The model under review builds one solid part; all positions refer to its coordinate system, in mm. A direction names the side the tool comes from. Give positions to 0.01 mm unless a question says otherwise; leave off trailing zeros. Order: outer loops, then holes, each group sorted by start corner. A loop starts at its lowest first (then second) coordinate and runs counter-clockwise, first axis right, second up. Notation, with made-up numbers: (-9.75, -30.5) - (6.25, -30.5) arc R18 cw to (6.25, -9.5) - close; hole circle Ø1 at (-7.5, 46). An arc over 180 degrees is marked (long way). Write item = value, one per line. Start each with the question number.
1. We need section A-A, the plane z = 0. Give the boundary of the cut face in (x, y), and give its area (3 significant figures).
2. Machinability: for faces 1 (the flat face through (-0.7, -2.1, 5.093)), 2 (the flat face through (-0.7, -2.1, -4.305)), which of the approach directions +Z, -Z, +X, -X, +Y, -Y give a long, thin tool a straight path to every point of the face, cutting with its end or side? Answer none if there is none.
3. For P1, Ø0.6, axis at x = 0, y = -2.5, coming from the -Z side; P2, Ø1, axis at x = 0.5, y = -2.5, coming from the +Z side; P3, Ø1, axis at x = 0.5, y = -2, coming from the -Z side; P4, Ø0.9, axis at x = 0, z = -4.5, coming from the -Y side, all flat-tipped, find the tip position at first contact; note any pin that passes through.
4. We need section C-C, the plane z = -4.5. Give the boundary of the cut face in (x, y).
5. We need section B-B, the plane y = -1.85. Give the boundary of the cut face in (x, z).
6. We need section D-D, the plane x = -1.75. Give the boundary of the cut face in (y, z), and give its area (3 significant figures).
7. Mouldability with a two-part tool opening along Z and no side actions: class faces 3 (the flat face through (0, 0, 1)), 4 (the flat face through (0, 0.254, 0)), 5 (the flat face through (-0.7, -2.1, -5.093)) as pulls with the +Z half, pulls with the -Z half, needs draft (parallel to the pull), parting line crosses it, or undercut.
8. Wall thickness on probe 1 along Z at (x, y) = (-0.75, -0.3); probe 2 along X at (y, z) = (-2.2, 4.75); probe 3 along Y at (x, z) = (-1.25, -5.25): over which ranges is each line inside the solid? List them lowest first.
Autodesk Inventor part; units mm, degrees
ref_plane "to_base_XY" through (0, 0, 0) normal (0, 1, 0) x (1, 0, 0)
ref_plane "to_base_YZ" through (0, 0, 0) normal (1, 0, 0) x (0, 0, -1)
ref_plane "to_base_ZX" through (0, 0, 0) normal (0, 0, -1) x (0, 1, 0)
sketch "Sketch_2" plane through (0, 0, 0) normal (0, 1, 0) x (-1, 0, 0)
  line L0 (3.1877, -6.1184) -> (3.1877, 6.1184)
  arc A0 (3.1877, 6.1184) -> (3.0577, 6.2484) centre (3.0577, 6.1184) ccw
  line L1 (3.0577, 6.2484) -> (-3.0577, 6.2484)
  arc A1 (-3.0577, 6.2484) -> (-3.1877, 6.1184) centre (-3.0577, 6.1184) ccw
  line L2 (-3.1877, 6.1184) -> (-3.1877, -6.1184)
  arc A2 (-3.1877, -6.1184) -> (-3.0577, -6.2484) centre (-3.0577, -6.1184) ccw
  line L3 (-3.0577, -6.2484) -> (3.0577, -6.2484)
  arc A3 (3.0577, -6.2484) -> (3.1877, -6.1184) centre (3.0577, -6.1184) ccw
extrude "Extrusion1" add sketch "Sketch_2" along normal blind 0.254
sketch "Sketch_1" plane through (0, 0, -4.699) normal (0, 0, 1) x (1, 0, 0)
  line L0 (-1.0033, 0) -> (-1.0033, -4.2418)
  line L1 (-1.0033, -4.2418) -> (1.0033, -4.2418)
  line L2 (1.0033, -4.2418) -> (1.0033, 0)
  line L3 (1.0033, 0) -> (-1.0033, 0)
  line L4 (-0.5461, -1.2446) -> (-0.5461, -3.2512)
  line L5 (-0.5461, -3.2512) -> (0.5461, -3.2512)
  line L6 (0.5461, -3.2512) -> (0.5461, -1.2446)
  line L7 (0.5461, -1.2446) -> (-0.5461, -1.2446)
extrude "Extrusion2" add sketch "Sketch_1" along normal mid plane 0.7874
pattern_linear "Rectangular Pattern1" count 2 spacing 9.398 along (0, 0, 1) of "Extrusion2"
sketch "Sketch_14" plane through (0, 0, 0) normal (0, 0, 1) x (1, 0, 0)
  line L0 (-1.0033, 0) -> (-1.0033, -4.7498)
  line L1 (-1.0033, -4.7498) -> (1.0033, -4.7498)
  line L2 (1.0033, -4.7498) -> (1.0033, 0)
  line L3 (1.0033, 0) -> (-1.0033, 0)
  line L4 (-0.5461, -1.4986) -> (-0.5461, -3.5052)
  line L5 (-0.5461, -3.5052) -> (0.5461, -3.5052)
  line L6 (0.5461, -3.5052) -> (0.5461, -1.4986)
  line L7 (0.5461, -1.4986) -> (-0.5461, -1.4986)
extrude "Extrusion3" add sketch "Sketch_14" along normal mid plane 0.7874
ref_plane "to_base_XY" through (0, 0, 0) normal (0, 1, 0) x (1, 0, 0)
ref_plane "to_base_YZ" through (0, 0, 0) normal (1, 0, 0) x (0, 0, -1)
ref_plane "to_base_ZX" through (0, 0, 0) normal (0, 0, -1) x (0, 1, 0)
properties part number "M201901-terminals"
Model answer:
q1.outline = (-3.19, 0) - (-1, 0) - (-1, -4.75) - (1, -4.75) - (1, 0) - (3.19, 0) - (3.19, 0.25) - (-3.19, 0.25) - close; hole (-0.55, -3.51) - (0.55, -3.51) - (0.55, -1.5) - (-0.55, -1.5) - close
q1.area = 8.96 mm2
q2.face_1 = +Z, +X, -X, -Y
q2.face_2 = +X, -X, -Y
q3.P1 = through
q3.P2 = 5.09
q3.P3 = -5.09
q3.P4 = -4.24
q4.outline = (-3.19, 0) - (-1, 0) - (-1, -4.24) - (1, -4.24) - (1, 0) - (3.19, 0) - (3.19, 0.25) - (-3.19, 0.25) - close; hole (-0.55, -3.25) - (0.55, -3.25) - (0.55, -1.24) - (-0.55, -1.24) - close
q5.outline = (-1, -5.09) - (-0.55, -5.09) - (-0.55, -4.31) - (-1, -4.31) - close; (-1, -0.39) - (-0.55, -0.39) - (-0.55, 0.39) - (-1, 0.39) - close; (-1, 4.31) - (-0.55, 4.31) - (-0.55, 5.09) - (-1, 5.09) - close; (0.55, -5.09) - (1, -5.09) - (1, -4.31) - (0.55, -4.31) - close; (0.55, -0.39) - (1, -0.39) - (1, 0.39) - (0.55, 0.39) - close; (0.55, 4.31) - (1, 4.31) - (1, 5.09) - (0.55, 5.09) - close
q6.outline = (0, -6.25) - (0.25, -6.25) - (0.25, 6.25) - (0, 6.25) - close
q6.area = 3.17 mm2
q7.face_3 = undercut
q7.face_4 = needs draft
q7.face_5 = pulls with the -Z half
q8.probe_1 = -5.09 to -4.31, -0.39 to 0.39, 4.31 to 5.09
q8.probe_2 = -1 to -0.55, 0.55 to 1
q8.probe_3 = 0 to 0.25
